Read the model definition and answer for the solid it produces. Units are mm, in the model's axes. Face numbers are marked on the shaded views. A direction names the side the tool comes from. Coordinates: 2 decimals unless noted, no trailing zeros. Write each loop counter-clockwise with the first axis right and the second up, starting at its lowest first coordinate (ties: lowest second). Pieces come first, ordered by that corner, then holes.
Item 1: Each of these flat-tipped pins is pushed along its axis until it touches: P1, Ø12, axis at y = 19.5, z = 23.5, coming from the -X side; P2, Ø4.5, axis at x = -24.5, z = 36.35, coming from the +Y side; P3, Ø3.5, axis at x = 31.5, y = 16.5, coming from the -Z side; P4, Ø3.5, axis at x = 30, z = 11, coming from the -Y side. Where does it stop, or does it pass through?
Item 2: Section C-C (z = 30) is taken. Give the vertices of the cut face in (x, y), then the cut area to 3 significant figures.
Item 3: A tool of negligible diameter and unlimited length cuts with its end or side. For the marked faces 1, 2, 3 and 4, from which of +Z, -Z, +X, -X, +Y, -Y can it reach the whole face along a straight path? Write none if from no direction.
Item 4: Straight lines are drawn through the part: probe 1 along Z at (x, y) = (24.5, 8.2) (3 decimals); probe 2 along Y at (x, z) = (32, 33.5); probe 3 along X at (y, z) = (19.5, -23). For each, find the intervals that lie inside material, in ascending order.
Item 5: Section D-D (y = 48.5) is taken. State how many separate pieces and enclosed holes the cut face has, then the cut area to 3 significant figures.
Item 6: Determine the mould class of the marked faces 5, 6 and 7 for opening direction Z: released by +Z, released by -Z, zero draft, split by the parting line, or undercut.
Item 7: Section A-A (z = 15.5) is taken. Give the vertices of the cut face in (x, y).
Item 8: Section B-B (x = 24.5) is taken. Give the vertices of the cut face in (y, z) (3 decimals), then the cut area to 3 significant figures.
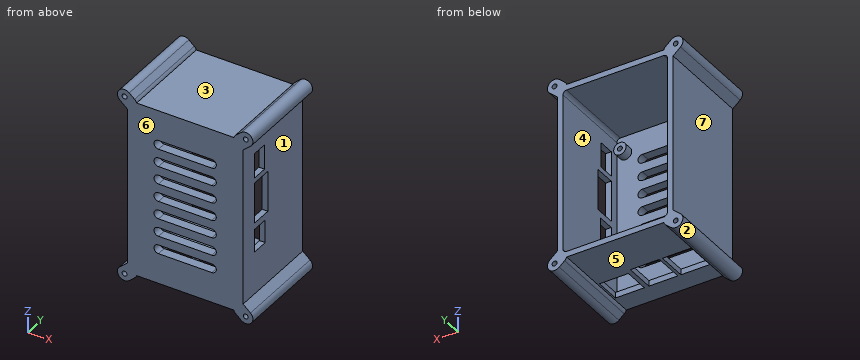
Autodesk Inventor part; units mm, degrees
ref_plane "YZ Plane" through (0, 0, 0) normal (1, 0, 0) x (0, 1, 0)
ref_plane "XZ Plane" through (0, 0, 0) normal (0, 1, 0) x (-1, 0, 0)
ref_plane "XY Plane" through (0, 0, 0) normal (0, 0, 1) x (1, 0, 0)
sketch "Sketch1" plane through (0, 0, 0) normal (0, 1, 0) x (-1, 0, 0)
  line L0 (-32.55, -49.55) -> (32.55, -49.55)
  line L1 (32.55, -49.55) -> (32.55, 49.55)
  line L2 (32.55, 49.55) -> (-32.55, 49.55)
  line L3 (-32.55, 49.55) -> (-32.55, -49.55)
  line L4 (-32.55, -49.55) -> (32.55, 49.55) construction
  line L5 (32.55, -49.55) -> (-32.55, 49.55) construction
  point P0 (0, 0)
  dimension "d0" = 65.1
  dimension "d1" = 99.1
extrude "Extrusion1" add sketch "Sketch1" along normal blind 5.08
sketch "Sketch2" plane through (0, 5.08, 0) normal (0, 1, 0) x (1, 0, 0)
  line L0 (29.35, 46.35) -> (-29.35, 46.35)
  line L1 (-29.35, 46.35) -> (-29.35, -46.35)
  line L2 (-29.35, -46.35) -> (29.35, -46.35)
  line L3 (29.35, -46.35) -> (29.35, 46.35)
  line L4 (29.35, 46.35) -> (-29.35, -46.35) construction
  line L5 (-29.35, 46.35) -> (29.35, -46.35) construction
  line L6 (-32.55, 49.55) -> (-32.55, -49.55)
  line L7 (-32.55, -49.55) -> (32.55, -49.55)
  line L8 (32.55, 49.55) -> (-32.55, 49.55)
  line L9 (32.55, -49.55) -> (32.55, 49.55)
  line L10 (26.15, -43.15) -> (32.55, -49.55) construction
  line L11 (23.6931, -46.35) -> (29.7216, -52.3784)
  line L12 (35.3784, -46.7216) -> (29.35, -40.6931)
  arc A0 (29.7216, -52.3784) -> (35.3784, -46.7216) centre (32.55, -49.55) ccw
  circle A1 centre (32.55, -49.55) radius 1.375
  point P0 (0, 0)
  dimension "d4" = 3.2
  dimension "d5" = 3.2
  dimension "d22" = 8
  dimension "d23" = 2.75
extrude "Extrusion2" add sketch "Sketch2" along normal blind 48 contours L0 L1 L2 L11 L7 L6 L8 L9 L12 L3 | L12 L9 A1 L7 L11 L2 L3 | L9 L7 A1 picked at (32.448, -48.6448)
sketch "Sketch3" plane through (0, 5.08, 0) normal (0, 1, 0) x (1, 0, 0)
  line L0 (29.35, -46.35) -> (-29.35, -46.35) construction
  line L1 (0, -46.35) -> (0, 46.35) construction
  line L2 (29.35, 46.35) -> (-29.35, 46.35) construction
  circle A0 centre (-24.5, -36.35) radius 3.5
  circle A1 centre (-24.5, -36.35) radius 1.375
  line L3 (29.35, 46.35) -> (29.35, -46.35) construction
  line L4 (29.35, 0) -> (-29.35, 0) construction
  line L5 (-29.35, -46.35) -> (-29.35, 46.35) construction
  circle A2 centre (-24.5, 21.65) radius 3.5
  circle A3 centre (-24.5, 21.65) radius 1.375
  circle A4 centre (24.5, -36.35) radius 3.5
  circle A5 centre (24.5, -36.35) radius 1.375
  circle A6 centre (24.5, 21.65) radius 3.5
  circle A7 centre (24.5, 21.65) radius 1.375
  point P0 (0, 0)
  dimension "d8" = 7
  dimension "d9" = 2.75
  dimension "d10" = 10
  dimension "d11" = 24.5
  dimension "d14" = 58
extrude "Extrusion3" add sketch "Sketch3" along normal blind 5
sketch "Sketch4" plane through (0, 0, 0) normal (0, -1, 0) x (1, 0, 0)
  line L0 (31.0438, 48.2342) -> (34.0562, 50.8658) construction
  line L1 (32.55, 49.55) -> (32.55, -49.55)
  line L2 (32.55, 44.2386) -> (36.6878, 47.8534)
  line L3 (31.4245, 53.8782) -> (28.4122, 51.2466)
  arc A0 (28.4122, 51.2466) -> (27.2664, 49.55) centre (31.0438, 48.2342) ccw
  arc A1 (36.6878, 47.8534) -> (31.4245, 53.8782) centre (34.0562, 50.8658) ccw
  line L4 (-32.55, 49.55) -> (32.55, 49.55)
  line L5 (27.2664, 49.55) -> (32.55, 49.55)
  line L6 (32.55, 49.55) -> (32.55, 44.2386)
  circle A2 centre (34.0562, 50.8658) radius 1.375
  line L7 (0, 49.55) -> (0, -49.55) construction
  line L8 (32.55, -49.55) -> (-32.55, -49.55) construction
  line L9 (32.55, 0) -> (-33.3, 0) construction
  line L10 (32.55, -49.55) -> (32.55, 49.55)
  line L11 (32.55, -44.2386) -> (36.6878, -47.8534)
  line L12 (31.4245, -53.8782) -> (28.4122, -51.2466)
  arc A3 (27.2664, -49.55) -> (28.4122, -51.2466) centre (31.0438, -48.2342) ccw
  arc A4 (31.4245, -53.8782) -> (36.6878, -47.8534) centre (34.0562, -50.8658) ccw
  line L13 (-32.55, -49.55) -> (32.55, -49.55)
  circle A5 centre (34.0562, -50.8658) radius 1.375
  line L14 (-32.55, 49.55) -> (-32.55, -49.55)
  line L15 (-32.55, 44.2386) -> (-36.6878, 47.8534)
  line L16 (-31.4245, 53.8782) -> (-28.4122, 51.2466)
  arc A6 (-27.2664, 49.55) -> (-28.4122, 51.2466) centre (-31.0438, 48.2342) ccw
  arc A7 (-31.4245, 53.8782) -> (-36.6878, 47.8534) centre (-34.0562, 50.8658) ccw
  line L17 (-27.2664, 49.55) -> (-32.55, 49.55)
  circle A8 centre (-34.0562, 50.8658) radius 1.375
  arc A9 (-36.6878, -47.8534) -> (-31.4245, -53.8782) centre (-34.0562, -50.8658) ccw
  line L18 (-32.55, -44.2386) -> (-36.6878, -47.8534)
  line L19 (-31.4245, -53.8782) -> (-28.4122, -51.2466)
  arc A10 (-28.4122, -51.2466) -> (-27.2664, -49.55) centre (-31.0438, -48.2342) ccw
  circle A11 centre (-34.0562, -50.8658) radius 1.375
  line L20 (-27.2664, -49.55) -> (-32.55, -49.55)
  line L21 (-32.55, -49.55) -> (-32.55, 49.55)
  point P0 (0, 0)
  point P1 (-32.55, -44.2386)
  point P2 (-27.2664, 49.55)
  point P3 (32.55, -49.55)
  dimension "d24" = 2
  dimension "d25" = 8
  dimension "d26" = 131.141
  dimension "d27" = 2.75
extrude "Extrusion4" add sketch "Sketch4" against normal up to surface (53.08 mm away) contours L4 A0 L3 A1 L2 L1 | L11 A4 L12 A3 L13 L1 | L4 L14 L15 A7 L16 A6 | A10 L19 A9 L18 L14 L13
fillet "Fillet2" radius 2 4 edges at (29.35, 29.08, -46.35) (-29.35, 29.08, -46.35) (-29.35, 29.08, 46.35) (29.35, 29.08, 46.35)
sketch "Sketch5" plane through (0, 5.08, 0) normal (0, 1, 0) x (1, 0, 0)
  line L0 (15, 0) -> (-15, 0) construction
  line L1 (15, 2.5) -> (-15, 2.5)
  line L2 (-15, -2.5) -> (15, -2.5)
  arc A0 (15, -2.5) -> (15, 2.5) centre (15, 0) ccw
  arc A1 (-15, 2.5) -> (-15, -2.5) centre (-15, 0) ccw
  line L3 (-27.35, -46.35) -> (27.35, -46.35) construction
  line L4 (0, -46.35) -> (0, 46.35) construction
  line L5 (-27.35, 46.35) -> (27.35, 46.35) construction
  arc A2 (-15, 12.5) -> (-15, 7.5) centre (-15, 10) ccw
  line L6 (15, 12.5) -> (-15, 12.5)
  line L7 (-15, 7.5) -> (15, 7.5)
  arc A3 (15, 7.5) -> (15, 12.5) centre (15, 10) ccw
  arc A4 (-15, 22.5) -> (-15, 17.5) centre (-15, 20) ccw
  line L8 (15, 22.5) -> (-15, 22.5)
  line L9 (-15, 17.5) -> (15, 17.5)
  arc A5 (15, 17.5) -> (15, 22.5) centre (15, 20) ccw
  arc A6 (-15, 32.5) -> (-15, 27.5) centre (-15, 30) ccw
  line L10 (15, 32.5) -> (-15, 32.5)
  line L11 (-15, 27.5) -> (15, 27.5)
  arc A7 (15, 27.5) -> (15, 32.5) centre (15, 30) ccw
  arc A8 (-15, -7.5) -> (-15, -12.5) centre (-15, -10) ccw
  line L12 (-15, -12.5) -> (15, -12.5)
  line L13 (15, -7.5) -> (-15, -7.5)
  arc A9 (15, -12.5) -> (15, -7.5) centre (15, -10) ccw
  arc A10 (-15, -17.5) -> (-15, -22.5) centre (-15, -20) ccw
  line L14 (-15, -22.5) -> (15, -22.5)
  line L15 (15, -17.5) -> (-15, -17.5)
  arc A11 (15, -22.5) -> (15, -17.5) centre (15, -20) ccw
  arc A12 (-15, -27.5) -> (-15, -32.5) centre (-15, -30) ccw
  line L16 (-15, -32.5) -> (15, -32.5)
  line L17 (15, -27.5) -> (-15, -27.5)
  arc A13 (15, -32.5) -> (15, -27.5) centre (15, -30) ccw
  point P0 (0, 0)
  dimension "d31" = 15
  dimension "d32" = 5
  dimension "d35" = 10
  dimension "d42" = 10
extrude "Extrusion5" cut sketch "Sketch5" against normal up to surface (5.08 mm away)
sketch "Sketch9" plane through (27.2664, 0, -49.55) normal (0, 0, -1) x (-1, 0, 0)
  line L0 (6.2664, 10.08) -> (-0.7336, 10.08)
  line L1 (1.3914, 10.08) -> (4.1414, 10.08)
  line L2 (1.3914, 10.08) -> (4.1414, 10.08) construction
  line L3 (2.7664, 10.08) -> (-0.7336, 10.08) construction
  line L4 (6.2664, 10.08) -> (-0.7336, 10.08)
  line L5 (0, 53.08) -> (0, 0)
  line L6 (-0.7336, 10.08) -> (0, 13.5023) construction
  line L7 (17.325, 11.35) -> (1.075, 11.35)
  line L8 (1.075, 11.35) -> (1.075, 25.6)
  line L9 (1.075, 25.6) -> (17.325, 25.6)
  line L10 (17.325, 25.6) -> (17.325, 11.35)
  line L11 (9.2, 25.6) -> (9.2, 11.35) construction
  line L12 (19.875, 11.35) -> (36.125, 11.35)
  line L13 (36.125, 11.35) -> (36.125, 27.85)
  line L14 (36.125, 27.85) -> (19.875, 27.85)
  line L15 (19.875, 27.85) -> (19.875, 11.35)
  line L16 (28, 27.85) -> (28, 11.35) construction
  line L17 (54.125, 27.85) -> (37.875, 27.85)
  line L18 (54.125, 11.35) -> (54.125, 27.85)
  line L19 (37.875, 11.35) -> (54.125, 11.35)
  line L20 (37.875, 27.85) -> (37.875, 11.35)
  point P0 (27.2664, 0)
  point P1 (46, 27.85)
  point P2 (46, 11.35)
  dimension "d58" = 3.5
  dimension "d60" = 3.5
  dimension "d63" = 16.25
  dimension "d64" = 14.25
  dimension "d65" = 1.27
  dimension "d66" = 9.2
  dimension "d69" = 16.25
  dimension "d70" = 16.5
  dimension "d71" = 1.27
  dimension "d72" = 28
  dimension "d75" = 18
extrude "Extrusion7" cut sketch "Sketch9" against normal up to surface (3.2 mm away)
sketch "Sketch12" plane through (32.55, 0, 44.2386) normal (1, 0, 0) x (0, 0, -1)
  line L0 (0, 53.08) -> (0, 0)
  line L1 (28.8305, 16.69) -> (28.8305, 14.2116)
  line L2 (43.8305, 14.2116) -> (43.8305, 16.69)
  line L3 (10.9402, 12.8971) -> (10.9402, 13.09)
  line L4 (18.9209, 13.09) -> (18.9209, 12.8971)
  line L5 (54.4305, 17.41) -> (54.4305, 11.41)
  line L6 (61.4305, 11.41) -> (61.4305, 17.41)
  line L7 (11.9305, 14.1354) -> (17.9305, 14.1354)
  line L8 (21.7386, 5.08) -> (26.7386, 5.08)
  line L9 (26.7386, 5.08) -> (21.7386, 5.08)
  line L10 (41.7386, 5.08) -> (46.7386, 5.08)
  line L11 (46.7386, 5.08) -> (41.7386, 5.08)
  line L12 (51.7386, 5.08) -> (56.7386, 5.08)
  line L13 (56.7386, 5.08) -> (51.7386, 5.08)
  line L14 (61.7386, 5.08) -> (66.7386, 5.08)
  line L15 (66.7386, 5.08) -> (61.7386, 5.08)
  line L16 (11.7386, 5.08) -> (16.7386, 5.08)
  line L17 (16.7386, 5.08) -> (11.7386, 5.08)
  line L18 (31.7386, 5.08) -> (36.7386, 5.08)
  line L19 (36.7386, 5.08) -> (31.7386, 5.08)
  line L20 (71.7386, 5.08) -> (76.7386, 5.08)
  line L21 (76.7386, 5.08) -> (71.7386, 5.08)
  line L22 (4.3886, 5.08) -> (11.3886, 5.08)
  line L23 (4.3886, 5.08) -> (11.3886, 5.08)
  line L24 (62.3886, 5.08) -> (69.3886, 5.08)
  line L25 (62.3886, 5.08) -> (69.3886, 5.08)
  line L26 (-2.1114, 5.08) -> (-0.1114, 5.08)
  line L27 (-0.1114, 5.08) -> (88.5886, 5.08)
  line L28 (88.5886, 5.08) -> (90.5886, 5.08)
  line L29 (90.5886, 5.08) -> (88.5886, 5.08)
  line L30 (88.5886, 5.08) -> (-0.1114, 5.08)
  line L31 (-0.1114, 5.08) -> (-2.1114, 5.08)
  line L32 (6.5136, 10.08) -> (9.2636, 10.08)
  line L33 (10.9402, 12.9936) -> (18.9209, 12.9936) construction
  line L34 (14.9305, 14.1354) -> (14.9305, 12.9936) construction
  line L35 (7.9402, 19.08) -> (21.9209, 19.08)
  line L36 (21.9209, 19.08) -> (21.9209, 10.08)
  line L37 (21.9209, 10.08) -> (7.9402, 10.08)
  line L38 (7.9402, 10.08) -> (7.9402, 19.08)
  line L39 (43.0305, 17.49) -> (29.6305, 17.49)
  line L40 (47.8305, 10.08) -> (24.8305, 10.08)
  line L41 (24.8305, 10.08) -> (24.8305, 22.08)
  line L42 (24.8305, 22.08) -> (47.8305, 22.08)
  line L43 (47.8305, 22.08) -> (47.8305, 10.08)
  line L44 (61.4305, 17.41) -> (57.9305, 17.41)
  line L45 (64.4305, 10.08) -> (51.4305, 10.08)
  line L46 (51.4305, 10.08) -> (51.4305, 19.68)
  line L47 (51.4305, 19.68) -> (64.4305, 19.68)
  line L48 (64.4305, 19.68) -> (64.4305, 10.08)
  point P0 (44.2386, 0)
  dimension "d99" = 3
  dimension "d100" = 3
  dimension "d101" = 0
  dimension "d102" = 9
  dimension "d103" = 4
  dimension "d104" = 4
  dimension "d105" = 0
  dimension "d106" = 12
  dimension "d108" = 3
  dimension "d109" = 3
  dimension "d110" = 0
  dimension "d111" = 9.6
extrude "Extrusion9" cut sketch "Sketch12" against normal up to surface (3.2 mm away)
properties part number "Case RevC" material "ABS Plastic"
Established:
1. P1: stops at x = -32.55
1. P2: stops at y = 10.08
1. P3: stops at z = -54.78
1. P4: stops at y = 0
2. outline: (-32.55, 0) - (-17.5, 0) - (-17.5, 5.08) - (-29.35, 5.08) - (-29.35, 53.08) - (-32.55, 53.08) - close; (17.5, 0) - (32.55, 0) - (32.55, 10.08) - (29.35, 10.08) - (29.35, 5.08) - (17.5, 5.08) - close; (29.35, 19.08) - (32.55, 19.08) - (32.55, 53.08) - (29.35, 53.08) - close
2. area: 431 mm2
3. face 1: +X, +Y, -Y
3. face 2: +Y, -Y
3. face 3: +Z, +Y, -Y
3. face 4: +Y
4. probe 1: z = -49.55 to -46.35, -25.15 to -23.025, -20.275 to -18.15, 32.85 to 34.975, 37.725 to 39.85, 46.35 to 49.55
4. probe 2: y = 0 to 10.08, 19.08 to 53.08
4. probe 3: x = -32.55 to -29.35, 29.35 to 32.55
5. separate pieces: 1
5. enclosed holes: 5
5. area: 1,220 mm2
6. face 5: released by -Z
6. face 6: zero draft
6. face 7: undercut
7. outline: (-32.55, 0) - (32.55, 0) - (32.55, 10.08) - (29.35, 10.08) - (29.35, 5.08) - (-29.35, 5.08) - (-29.35, 53.08) - (-32.55, 53.08) - close; (29.35, 22.08) - (32.55, 22.08) - (32.55, 53.08) - (29.35, 53.08) - close
8. outline: (0, -49.55) - (11.35, -49.55) - (11.35, -46.35) - (5.08, -46.35) - (5.08, -25.15) - (10.08, -25.15) - (10.08, -23.025) - (5.08, -23.025) - (5.08, -20.275) - (10.08, -20.275) - (10.08, -18.15) - (5.08, -18.15) - (5.08, 32.85) - (10.08, 32.85) - (10.08, 34.975) - (5.08, 34.975) - (5.08, 37.725) - (10.08, 37.725) - (10.08, 39.85) - (5.08, 39.85) - (5.08, 46.35) - (53.08, 46.35) - (53.08, 49.55) - (0, 49.55) - close; (25.6, -49.55) - (53.08, -49.55) - (53.08, -46.35) - (25.6, -46.35) - close
8. area: 808 mm2
